from build123d import *

# Parameters (mm, degrees)
F0_W        = 17.6611579955
F0_H        = 5.08
F1_DEPTH    = 5.08
F2_T1_DEPTH = 55.76598658
F2_T3_DEPTH = 24.0135722877
F4_DEPTH    = 5.081
F6_DEPTH    = 2.54


# Not quite as in the source:
# - a fillet or chamfer that OpenCascade refuses, or shapes differently, is made with other operations: its cross-section is extruded or revolved along the edge and cut away or added


with BuildPart() as f1:
    # F0 (on Top) → F1 (new body)
    with BuildSketch(Plane.XY):
        with Locations((-8.8305789977, 2.54)):
            Rectangle(F0_W, F0_H)
        Polygon((0, 5.08), (0, 0), (25.4, 0), (25.4, 31.75), (88.9, 31.75), (114.3, 31.75), (114.3, 63.5), (0, 63.5), (0, 28.7528), align=None)
    extrude(amount=F1_DEPTH)

    # F2: fillet of radius 2.54 on 4 edges, made by hand

    # F2_s2 → F2_t1 (cut)
    with BuildSketch(Plane.YZ.offset(-24.0135722877)):
        with BuildLine():
            ThreePointArc((-0.0004, 2.5390343146), (0.7439487758, 4.3360512242), (2.5409656854, 5.0804))
            Line((2.5409656854, 5.0804), (2.5409656854, 5.3345365685))
            ThreePointArc((2.5409656854, 5.3345365685), (1.2704828427, 5.3341365685), (0, 5.3341365685))
            Line((0, 5.3341365685), (-0.2541365685, 5.08))
            ThreePointArc((-0.2541365685, 5.08), (-0.2541365685, 3.8095171573), (-0.2545365685, 2.5390343146))
            Line((-0.2545365685, 2.5390343146), (-0.0004, 2.5390343146))
        make_face()
        with BuildLine():
            ThreePointArc((-0.0004, 2.5409656854), (0.7439487758, 0.7439487758), (2.5409656854, -0.0004))
            Line((2.5409656854, -0.0004), (2.5409656854, -0.2545365685))
            ThreePointArc((2.5409656854, -0.2545365685), (1.2704828427, -0.2541365685), (0, -0.2541365685))
            Line((0, -0.2541365685), (-0.2541365685, 0))
            ThreePointArc((-0.2541365685, 0), (-0.2541365685, 1.2704828427), (-0.2545365685, 2.5409656854))
            Line((-0.2545365685, 2.5409656854), (-0.0004, 2.5409656854))
        make_face()
    extrude(amount=F2_T1_DEPTH, mode=Mode.SUBTRACT)

    # F2_s4 → F2_t3 (cut)
    with BuildSketch(Plane.YZ.offset(-24.0135722877)):
        with BuildLine():
            ThreePointArc((5.0804, 2.5390343146), (4.3360512242, 4.3360512242), (2.5390343146, 5.0804))
            Line((2.5390343146, 5.0804), (2.5390343146, 5.3345365685))
            ThreePointArc((2.5390343146, 5.3345365685), (3.8095171573, 5.3341365685), (5.08, 5.3341365685))
            Line((5.08, 5.3341365685), (5.3341365685, 5.08))
            ThreePointArc((5.3341365685, 5.08), (5.3341365685, 3.8095171573), (5.3345365685, 2.5390343146))
            Line((5.3345365685, 2.5390343146), (5.0804, 2.5390343146))
        make_face()
        with BuildLine():
            ThreePointArc((5.0804, 2.5409656854), (4.3360512242, 0.7439487758), (2.5390343146, -0.0004))
            Line((2.5390343146, -0.0004), (2.5390343146, -0.2545365685))
            ThreePointArc((2.5390343146, -0.2545365685), (3.8095171573, -0.2541365685), (5.08, -0.2541365685))
            Line((5.08, -0.2541365685), (5.3341365685, 0))
            ThreePointArc((5.3341365685, 0), (5.3341365685, 1.2704828427), (5.3345365685, 2.5409656854))
            Line((5.3345365685, 2.5409656854), (5.0804, 2.5409656854))
        make_face()
    extrude(amount=F2_T3_DEPTH, mode=Mode.SUBTRACT)

    # F3 (on face) → F4 (cut, through all)
    with BuildSketch(Plane.XY.offset(5.08)):
        with BuildLine():
            ThreePointArc((-7.7692847717, 2.54), (-8.89, 3.6607152283), (-10.0107152283, 2.54))
            Line((-10.0107152283, 2.54), (-7.7692847717, 2.54))
        make_face()
        with BuildLine():
            Line((-7.7692847717, 2.54), (-10.0107152283, 2.54))
            ThreePointArc((-10.0107152283, 2.54), (-8.89, 1.4192847717), (-7.7692847717, 2.54))
        make_face()
    extrude(amount=-F4_DEPTH, mode=Mode.SUBTRACT)

    # F5 (on face) → F6 (join)
    with BuildSketch(Plane(origin=(0, 0, 0), x_dir=(0, -1, 0), z_dir=(-1, 0, 0))):
        with BuildLine():
            Line((-2.54, 2.54), (-2.54, 6.35))
            ThreePointArc((-2.54, 6.35), (-4.0954259867, 6.0180382402), (-5.3798063314, 5.08))
            Line((-5.3798063314, 5.08), (-2.5841223678, 5.08))
            ThreePointArc((-2.5841223678, 5.08), (-4.3360512242, 4.3360512242), (-5.08, 2.5841223678))
            Line((-5.08, 2.5841223678), (-5.08, 2.54))
            Line((-5.08, 2.54), (-2.54, 2.54))
        make_face()
        with BuildLine():
            ThreePointArc((-6.35, 2.54), (-6.0991966876, 1.180507838), (-5.3798063314, 0))
            Line((-5.3798063314, 0), (-2.5841223678, 0))
            ThreePointArc((-2.5841223678, 0), (-4.3360512242, 0.7439487758), (-5.08, 2.4958776322))
            Line((-5.08, 2.4958776322), (-5.08, 2.54))
            Line((-5.08, 2.54), (-6.35, 2.54))
        make_face()
        with BuildLine():
            Line((-2.5841223678, 5.08), (-5.3798063314, 5.08))
            ThreePointArc((-5.3798063314, 5.08), (-6.0991966876, 3.899492162), (-6.35, 2.54))
            Line((-6.35, 2.54), (-5.08, 2.54))
            Line((-5.08, 2.54), (-5.08, 2.5841223678))
            ThreePointArc((-5.08, 2.5841223678), (-4.3360512242, 4.3360512242), (-2.5841223678, 5.08))
        make_face()
        with BuildLine():
            Line((-2.54, 0), (-2.54, 2.54))
            Line((-2.54, 2.54), (-5.08, 2.54))
            Line((-5.08, 2.54), (-5.08, 2.4958776322))
            ThreePointArc((-5.08, 2.4958776322), (-4.3360512242, 0.7439487758), (-2.5841223678, 0))
            Line((-2.5841223678, 0), (-2.54, 0))
        make_face()
    extrude(amount=F6_DEPTH)


solid = f1.part
The model under review builds one solid part; all positions refer to its coordinate system, in mm. A direction names the side the tool comes from. Round coordinates to 2 decimals unless told otherwise and drop trailing zeros. Order: outer loops, then holes, each group sorted by start corner. A loop starts at its lowest first (then second) coordinate and runs counter-clockwise, first axis right, second up. Notation, with made-up numbers: (5, -14) -> (39, -14) arc R14 cw to (39, 11) -> close; hole circle Ø8 at (83, -40). An arc over 180 degrees is marked (long way). Write item = value, one per line. Start each with the question number.
Item 1: Consider section D-D on y = 24.5. Write out the cut boundary in (x, z).
Item 2: Clearance check with flat-ended pins moving along their axes: pin 1 Ø3 at (x, y) = (-8.89, 2.54) entering from +Z; pin 2 Ø1.5 at (y, z) = (47.5, 4) entering from -X; pin 3 Ø3 at (x, z) = (40.5, 4.5) entering from -Y. State where each tip first meets the part, or that it passes through.
Item 3: Consider section C-C on y = 58. Write out the cut boundary in (x, z).
Item 4: Consider section A-A on x = 9. Write out the cut boundary in (y, z).
Item 5: For line 1 along X through (y, z) = (2.54, 2.85); line 2 along X through (y, z) = (57, 4.75); line 3 along Y through (x, z) = (-8.89, 2.3), list the stretches that pass through material, from the lowest coordinate up.
Item 6: For faces 5 (the face through (-10.206, 4.355, 4.317)), 6 (the face through (-10.206, 4.355, 0.763)), 7 (the face through (25.4, 16, 3)), list the 3-axis set-ups (+Z, -Z, +X, -X, +Y, -Y) from which the entire face can be reached by the end or side of a thin tool; tool diameter is ignored.
Item 7: Consider section B-B on z = 1.5. Write out the cut boundary in (x, y), plus the area to 3 significant figures.
Item 8: Mouldability with a two-part tool opening along X and no side actions: class faces 1 (the face through (69, 31.75, 3)), 2 (the face through (-9.925, 2.969, 2.576)), 3 (the face through (114.3, 47, 3)), 4 (the face through (-2.54, 5.3, 3.2)) as released by +X, released by -X, zero draft, split by the parting line, or undercut.
Conclusion:
q1.outline = (0, 0) -> (25.4, 0) -> (25.4, 5.08) -> (0, 5.08) -> close
q2.pin_1 = 5.08
q2.pin_2 = 0
q2.pin_3 = 31.75
q3.outline = (0, 0) -> (114.3, 0) -> (114.3, 5.08) -> (0, 5.08) -> close
q4.outline = (0, 2.5) arc R2.54 ccw to (2.5, 0) -> (63.5, 0) -> (63.5, 5.08) -> (2.5, 5.08) arc R2.54 ccw to (0, 2.58) -> close
q5.line_1 = -17.66 to -10.01, -7.77 to 25.4
q5.line_2 = 0 to 114.3
q5.line_3 = 0.01 to 1.42, 3.66 to 5.07
q6.face_5 = +Z, -X, +Y
q6.face_6 = -Z, -X, +Y
q6.face_7 = +Z, -Z, +X, -Y
q7.outline = (-17.66, 0.22) -> (25.4, 0.22) -> (25.4, 31.75) -> (114.3, 31.75) -> (114.3, 63.5) -> (0, 63.5) -> (0, 6.21) -> (-2.54, 6.21) -> (-2.54, 4.86) -> (-17.66, 4.86) -> close; hole circle Ø2.24 at (-8.89, 2.54)
q7.area = 4,510 mm2
q8.face_1 = zero draft
q8.face_2 = undercut
q8.face_3 = released by +X
q8.face_4 = released by -X
